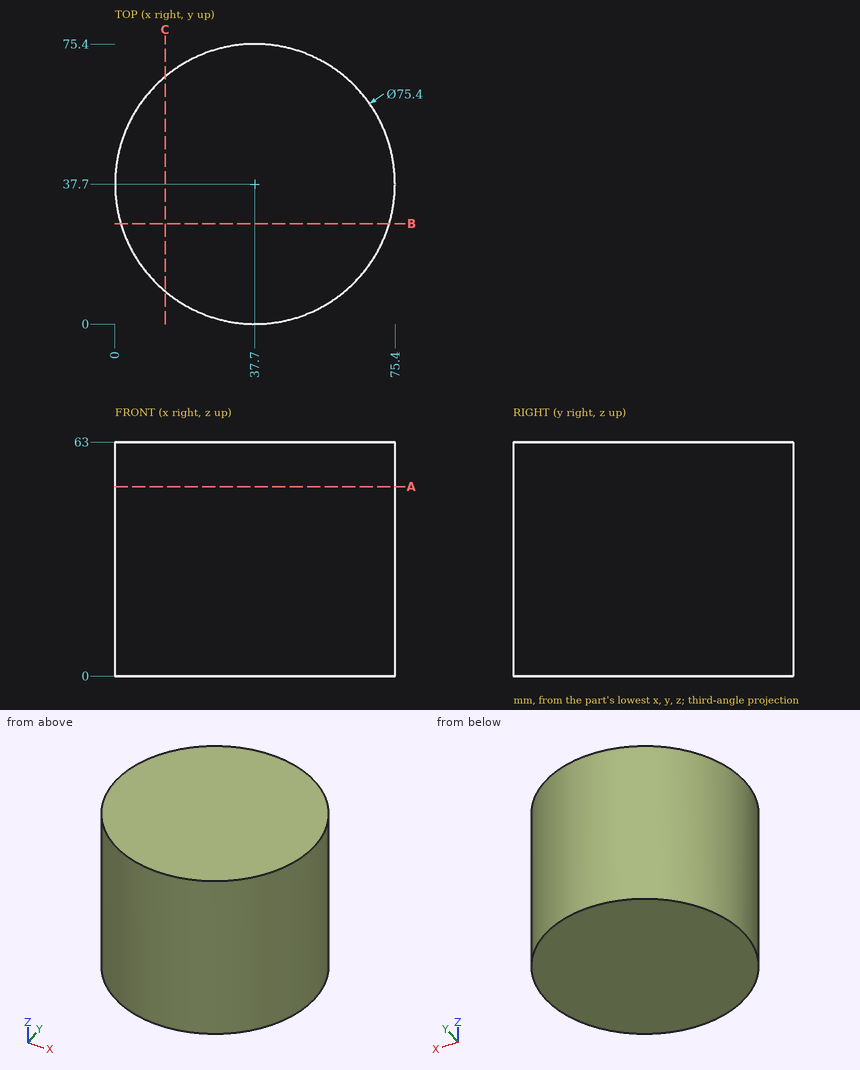
Verification items for this drawing (mm, ordinates from the low corner). Give positions to 0.01 mm unless a question says otherwise; leave off trailing zeros. Write each loop counter-clockwise with the first axis right and the second up, starting at its lowest first coordinate (ties: lowest second). Pieces come first, ordered by that corner, then holes. Notation, with made-up numbers: (56, 18.25) -> (61, 18.25) arc R25 cw to (61, 56.25) -> close; hole circle Ø11 at (-33, 11.5). An arc over 180 degrees is marked (long way). Write item = value, one per line.
Item 1: Sectioned sample at B-B on y = 27. Record the boundary of the cut face in (x, z), and give its area (3 significant figures).
Output:
outline = (1.55, 0) -> (73.85, 0) -> (73.85, 63) -> (1.55, 63) -> close
area = 4,550 mm^2
Item 2: Sectioned sample at C-C on x = 13.5. Record the boundary of the cut face in (y, z).
Output:
outline = (8.79, 0) -> (66.61, 0) -> (66.61, 63) -> (8.79, 63) -> close
Item 3: Sectioned sample at A-A on z = 51. Record the boundary of the cut face in (x, y), and give its area (3 significant figures).
Output:
outline = circle Ø75.4 at (37.7, 37.7)
area = 4,470 mm^2
Item 4: Gauge pin test, flat ends, axial feed: pin 1 (2 mm diameter, centred on y = 11.5, z = 12.5, fed in from -X); pin 2 (5 mm diameter, centred on x = 41, y = 64.5, fed in from -Z); pin 3 (3 mm diameter, centred on x = 22, z = 47, fed in from -Y); pin 4 (8 mm diameter, centred on x = 16, z = 56.5, fed in from +Y). Record the tip position at first contact, or that the pin passes through.
Output:
pin_1 = 9.66
pin_2 = 0
pin_3 = 2.78
pin_4 = 70.99
Item 5: Scan lines: probe 1 along X at (y, z) = (37.5, 45.5); probe 2 along Y at (x, z) = (65.5, 36); probe 3 along X at (y, z) = (63, 36). Record each from-to range of solid material in increasing order. Write a range as from..to.
Output:
probe_1 = 0..75.4
probe_2 = 12.24..63.16
probe_3 = 9.75..65.65
